Autodesk Inventor part; units mm, degrees
ref_plane "YZ Plane" through (0, 0, 0) normal (1, 0, 0) x (0, 1, 0)
ref_plane "XZ Plane" through (0, 0, 0) normal (0, 1, 0) x (-1, 0, 0)
ref_plane "XY Plane" through (0, 0, 0) normal (0, 0, 1) x (1, 0, 0)
sketch "Skizze1" plane through (0, 0, 0) normal (0, 0, 1) x (1, 0, 0)
  line L0 (-14.1284, 0) -> (-14.1284, 16.2)
  line L1 (-14.1284, 16.2) -> (-12.1284, 16.2)
  line L2 (-12.1284, 16.2) -> (-12.1284, 1.6)
  line L3 (-12.1284, 1.6) -> (12.3716, 1.6)
  line L4 (12.3716, 1.6) -> (12.3716, 16.2)
  line L5 (12.3716, 16.2) -> (14.3716, 16.2)
  line L6 (14.3716, 16.2) -> (14.3716, 0)
  line L7 (14.3716, 0) -> (-14.1284, 0)
  line L8 (-16.6284, 19.2) -> (19.3716, 19.2)
  line L9 (19.3716, 19.2) -> (19.3716, -3)
  line L10 (19.3716, -3) -> (-16.6284, -3)
  line L11 (-16.6284, -3) -> (-16.6284, 19.2)
  line L12 (-12.1284, 14.7) -> (12.3716, 14.7)
  point P0 (0, 0)
  dimension "d1" = 2
  dimension "d3" = 2
  dimension "d4" = 1.6
  dimension "d5" = 3
  dimension "d7" = 2.5
  dimension "d8" = 5
  dimension "d9" = 1.5
  dimension "d26" = 3
  dimension "d27" = 28.5
  dimension "d28" = 16.2
extrude "Extrusion1" add sketch "Skizze1" along normal blind 30
ref_plane "Arbeitsebene1" through (19.3716, -1, 28) normal (1, 0, 0) x (0, 0, -1)
sketch "Skizze5" plane through (19.3716, -1, 28) normal (1, 0, 0) x (0, 0, -1)
  circle A0 centre (13, 9.1) radius 2.4
  line L0 (13, 9.1) -> (-2, 9.1)
  line L1 (-2, 18.2) -> (-2, 0)
  line L2 (13, 9.1) -> (13, 20.2)
  line L3 (8, 20.2) -> (18, 20.2)
  line L4 (13, 9.1) -> (28, 9.1)
  point P0 (28, 1)
  dimension "d31" = 4.8
  dimension "d32" = 90
  dimension "d35" = 15
extrude "Extrusion5" cut sketch "Skizze5" against normal blind 10
sketch "Skizze6" plane through (-16.6284, 19.2, 0) normal (0, 1, 0) x (1, 0, 0)
  line L0 (36, -30) -> (0, -30)
  line L1 (36, -30) -> (26, -30)
  line L2 (26, -30) -> (26, 0)
  line L3 (26, 0) -> (36, 0)
  line L4 (36, 0) -> (36, -30)
  line L5 (0.0037, -30) -> (10.0037, -30)
  line L6 (10.0037, -30) -> (10.0037, 0)
  line L7 (10.0037, 0) -> (0.0037, 0)
  line L8 (0.0037, 0) -> (0.0037, -30)
  line L9 (26, -30) -> (36, -30)
  line L10 (36, -30) -> (36, -40)
  line L11 (36, -40) -> (26, -40)
  line L12 (26, -40) -> (26, -30)
  line L13 (26, 0) -> (36, 0)
  line L14 (36, 0) -> (36, 10)
  line L15 (36, 10) -> (26, 10)
  line L16 (26, 10) -> (26, 0)
  line L17 (0.0037, 0) -> (10.0037, 0)
  line L18 (10.0037, 0) -> (10.0037, 10)
  line L19 (10.0037, 10) -> (0.0037, 10)
  line L20 (0.0037, 10) -> (0.0037, 0)
  line L21 (0.0037, -30) -> (10.0037, -30)
  line L22 (10.0037, -30) -> (10.0037, -40)
  line L23 (10.0037, -40) -> (0.0037, -40)
  line L24 (0.0037, -40) -> (0.0037, -30)
  point P0 (16.6284, 0)
  dimension "d36" = 10
  dimension "d37" = 30
  dimension "d38" = 10
  dimension "d39" = 30
  dimension "d40" = 10
  dimension "d41" = 10
  dimension "d42" = 10
  dimension "d43" = 10
  dimension "d44" = 10
  dimension "d45" = 10
  dimension "d46" = 10
  dimension "d47" = 10
extrude "Extrusion7" add sketch "Skizze6" along normal blind 10
sketch "Skizze8" plane through (-16.6248, 19.2, 30) normal (-1, 0, 0) x (0, 0, 1)
  line L0 (-40, 0) -> (-40, 10)
  point P0 (-30, -19.2)
  point P1 (-27.5, 5)
  point P2 (-15, 5)
  point P3 (-2.5, 5)
  dimension "d52" = 12.5
  dimension "d53" = 12.5
  dimension "d54" = 12.5
hole "Bohrung1" at (-16.6248, 24.2, 2.5) at (-16.6248, 24.2, 15) at (-16.6248, 24.2, 27.5) direction (1, 0, 0) diameter 6.15 end through all
properties part number "Objektträgerhalter 2 6,15mm"
Geometry: final body of the model. Coordinates: model frame, mm. A direction names the side the tool comes from. Round coordinates to 2 decimals unless told otherwise and drop trailing zeros. Order: outer loops, then holes, each group sorted by start corner. A loop starts at its lowest first (then second) coordinate and runs counter-clockwise, first axis right, second up. Notation, with made-up numbers: (30.5, 44.25) - (37.5, 44.25) arc R17 cw to (37.5, 59.25) - close; hole circle Ø4 at (33, 73.25). An arc over 180 degrees is marked (long way). Use CSV: the item, a comma, the result in double quotes. Start each with the question number.
Q1. Section query B-B (z = 15). State how many separate pieces and enclosed holes the cut face has, and give its area (3 significant figures).
Q2. Access query for faces 4 (the face through (0, 0, 15)), 5 (the face through (-12, 19.2, -5)), 6 (the face through (-6.625, 27.5, 14.7)), 7 (the face through (14, 19.2, 35)). Directions: +Z, -Z, +X, -X, +Y, -Y. A direction counts if a zero-diameter tool reaches every point of the face in a straight line with its end or side. Return the directions, or none.
Q3. Material intervals for line 1 along Z through (x, y) = (13.75, 24.2) (3 decimals); line 2 along Y through (x, z) = (-12.5, 27.5) (3 decimals); line 3 along X through (y, z) = (4.5, 17), sorted ascending. Write a range as from..to.
Q4. First-contact query: pin 1 (8 mm diameter, centred on x = -11.5, z = -5.5, fed in from -Y); pin 2 (8 mm diameter, centred on x = 7, y = 3.5, fed in from +Z); pin 3 (3 mm diameter, centred on y = 23.5, z = 10.5, fed in from -X). Flat tips, straight axial feed; report the tip coordinate or a pass-through.
Q5. Mould query, pull axis X, two halves, no side actions, for faces 1 (the face through (-16.628, 8, 15)), 2 (the face through (0, 14.7, 15)), 3 (the face through (14.44, 21.15, 2.1)). Classes: +X half, -X half, draft (parallel to the pull), parting line (faces both ways), or undercut.
Q6. Section query A-A (x = -8.5). Return loops of the section in (y, z) (3 decimals), and give its area (3 significant figures).
Result set:
1,separate pieces,"3"
1,enclosed holes,"0"
1,area,"427 mm2"
2,face 4,"+Z, -Z"
2,face 5,"-Z, +X, -X, -Y"
2,face 6,"+Z, -Z, +Y"
2,face 7,"+Z, +X, -X, -Y"
3,line 1,"z = -10..-0.575, 5.575..11.925, 18.075..24.425, 30.575..40"
3,line 2,"y = -3..0, 16.2..21.125, 27.275..29.2"
3,line 3,"x = -16.63..-14.13, 14.37..19.37"
4,pin 1,"stops at y = 19.2"
4,pin 2,"stops at z = 30"
4,pin 3,"stops at x = -16.62"
5,face 1,"-X half"
5,face 2,"undercut"
5,face 3,"draft"
6,outline,"(-3, 0) - (0, 0) - (0, 30) - (-3, 30) - close; (14.7, 0) - (19.2, 0) - (19.2, -10) - (29.2, -10) - (29.2, 40) - (19.2, 40) - (19.2, 30) - (14.7, 30) - close; hole circle Ø6.15 at (24.2, 2.5); hole circle Ø6.15 at (24.2, 15); hole circle Ø6.15 at (24.2, 27.5)"
6,area,"636 mm2"
